```python
from build123d import *

# Parameters (mm, degrees)
F0_R     = 1.5
F0_W     = 210
F0_H     = 164
F1_DEPTH = 6


with BuildPart() as f1:
    # F0 (on Top) → F1 (new body)
    with BuildSketch(Plane.XY):
        with BuildLine():
            Line((-115, -92.5), (115, -92.5))
            ThreePointArc((115, -92.5), (118.535534, -91.035534), (120, -87.5))
            Line((120, -87.5), (120, 87.5))
            ThreePointArc((120, 87.5), (118.535534, 91.035534), (115, 92.5))
            Line((115, 92.5), (-115, 92.5))
            ThreePointArc((-115, 92.5), (-118.535534, 91.035534), (-120, 87.5))
            Line((-120, 87.5), (-120, -87.5))
            ThreePointArc((-120, -87.5), (-118.535534, -91.035534), (-115, -92.5))
        make_face()
        with Locations((-105.399, -87.9)):
            Circle(F0_R, mode=Mode.SUBTRACT)
        with Locations((-112.4, -52.4)):
            Circle(F0_R, mode=Mode.SUBTRACT)
        with Locations((105.399, -87.9)):
            Circle(F0_R, mode=Mode.SUBTRACT)
        with Locations((112.4, -52.4)):
            Circle(F0_R, mode=Mode.SUBTRACT)
        with Locations((-112.4, 52.4)):
            Circle(F0_R, mode=Mode.SUBTRACT)
        with Locations((-105.399, 87.9)):
            Circle(F0_R, mode=Mode.SUBTRACT)
        Rectangle(F0_W, F0_H, mode=Mode.SUBTRACT)
        with Locations((112.4, 52.4)):
            Circle(F0_R, mode=Mode.SUBTRACT)
        with Locations((105.399, 87.9)):
            Circle(F0_R, mode=Mode.SUBTRACT)
    extrude(amount=F1_DEPTH)


solid = f1.part
```
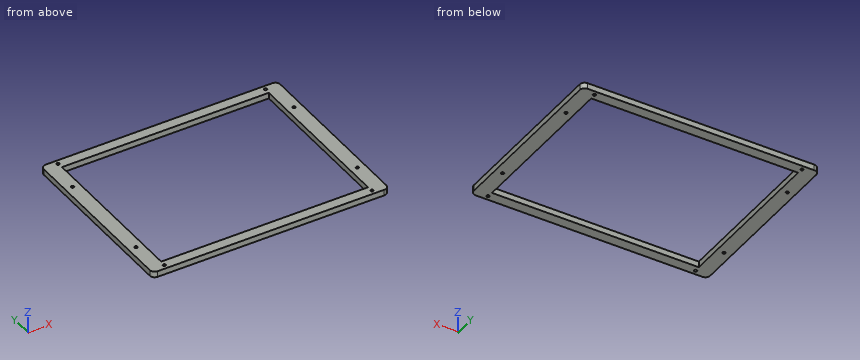
CAD build for the part. Positions are in the model's coordinates, mm. Coordinates: 2 decimals unless noted, no trailing zeros. Order: outer loops, then holes, each group sorted by start corner. A loop starts at its lowest first (then second) coordinate and runs counter-clockwise, first axis right, second up. Notation, with made-up numbers: (-3.5, 52) - (48.5, 52) arc R14 cw to (48.5, 65) - close; hole circle Ø6 at (-5, 1.5). An arc over 180 degrees is marked (long way). Use a Markdown table: item, result. Add a question column.
(1) Saw through at A-A (x = 62.5). Give the cut face in (y, z), then the cut area to 3 significant figures.
(2) Flat gauge pin, fed straight in: pin 1 (2.5 mm diameter, centred on x = 112.4, y = -52.4, fed in from -Z). Where does the tip first touch, or does it go through?
(3) Drill centre lines: line 1 along X through (y, z) = (-87.9, 4.2); line 2 along Y through (x, z) = (-112.4, 3.6); line 3 along Y through (x, z) = (-64, 4.3). Where is each one in solid material? Low to high. Write a range as [from, to].
(4) Saw through at B-B (y = -72.5). Give the cut face in (x, z).
(5) Saw through at C-C (z = 4.65). Count the separate pieces of the cut face and the enclosed holes in it, then the cut area to 3 significant figures.
Solved:
| question | item | result |
|---|---|---|
| 1 | outline | (-92.5, 0) - (-82, 0) - (-82, 6) - (-92.5, 6) - close; (82, 0) - (92.5, 0) - (92.5, 6) - (82, 6) - close |
| 1 | area | 126 mm² |
| 2 | pin 1 | passes through |
| 3 | line 1 | x = [-119.98, -106.9], [-103.9, 103.9], [106.9, 119.98] |
| 3 | line 2 | y = [-92.5, -53.9], [-50.9, 50.9], [53.9, 92.5] |
| 3 | line 3 | y = [-92.5, -82], [82, 92.5] |
| 4 | outline | (-120, 0) - (-105, 0) - (-105, 6) - (-120, 6) - close; (105, 0) - (120, 0) - (120, 6) - (105, 6) - close |
| 5 | separate pieces | 1 |
| 5 | enclosed holes | 9 |
| 5 | area | 9,880 mm² |
